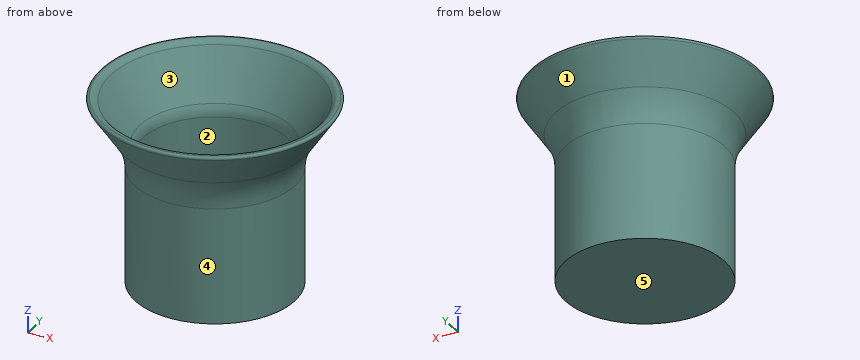
```python
from build123d import *


with BuildPart() as part:
    # Sketch → Revolution (revolve)
    with BuildSketch(Plane.XZ):
        with BuildLine():
            Line((0, 0), (-30, 0))
            Line((-30, 0), (-30, 43.518658))
            ThreePointArc((-30, 43.518658), (-30.926805, 49.716476), (-33.626135, 55.372051))
            Line((-33.626135, 55.372051), (-42.643328, 68.730856))
            ThreePointArc((-41.968787, 70), (-42.687419, 69.568119), (-42.643328, 68.730856))
            Line((-41.968787, 70), (-41.81553, 70))
            ThreePointArc((-39.010557, 68.47778), (-40.219831, 69.594921), (-41.81553, 70))
            Line((-39.010557, 68.47778), (-28.297456, 51.996087))
            ThreePointArc((-27, 47.619295), (-27.331193, 49.901821), (-28.297456, 51.996087))
            Line((-27, 12.91057), (-27, 47.619295))
            ThreePointArc((-27, 12.91057), (-24.243708, 6.256292), (-17.58943, 3.5))
            Line((0, 3.5), (-17.58943, 3.5))
            Line((0, 0), (0, 3.5))
        make_face()
    revolve(axis=Axis((0, 0, 0), (0, 0, 1)))


solid = part.part
```
Part model, mm, in its own coordinate system. Face numbers are marked on the shaded views. A direction names the side the tool comes from. Coordinates: 2 decimals unless noted, no trailing zeros. Order: outer loops, then holes, each group sorted by start corner. A loop starts at its lowest first (then second) coordinate and runs counter-clockwise, first axis right, second up. Notation, with made-up numbers: (28, -6) -> (83, -6) arc R24 ccw to (83, 27) -> close; hole circle Ø1 at (72.5, 41). An arc over 180 degrees is marked (long way). Put each result on its own line as item: value. Start each with the question number.
(1) Band-saw the part on D-D (z = 9.5). Give the cut face in (x, y), then the cut area to 3 significant figures.
(2) Which spindle directions (+Z, -Z, +X, -X, +Y, -Y) get a long thin tool onto all of the face, cutting with end or side? Do the marked faces 1 and 2. Say none if no direction does.
(3) Probe line 1 along X through (y, z) = (0, 25.5); line 2 along Y through (x, z) = (23.5, 65.5). List the from-to ranges inside material, lowest first. Write a range as [from, to].
(4) Band-saw the part on B-B (z = 26). Give the cut face in (x, y), then the cut area to 3 significant figures.
(5) Mould opens along Y. For the marked faces 3, 4 and 5 say: pulls with the +Y half, pulls with the -Y half, needs draft (parallel to the pull), parting line crosses it, or undercut.
(6) Band-saw the part on A-A (x = 0). Give the cut face in (y, z), then the cut area to 3 significant figures.
(7) Pin check, flat tips, straight feed: pin 1 Ø1 at (y, z) = (30, 58.5) entering from -X; pin 2 Ø6 at (x, z) = (-6.5, 45) entering from -Y; pin 3 Ø1 at (y, z) = (-26, 13) entering from +X. Stop position of each tip, or through.
Determined:
1. outline: circle Ø60 at (0, 0); hole circle Ø52.72 at (0, 0)
1. area: 644 mm²
2. face 1: -Z
2. face 2: +Z
3. line 1: x = [-30, -27], [27, 30]
3. line 2: y = [-32.94, -28.68], [28.68, 32.94]
4. outline: circle Ø60 at (0, 0); hole circle Ø54 at (0, 0)
4. area: 537 mm²
5. face 3: undercut
5. face 4: parting line crosses it
5. face 5: needs draft
6. outline: (-42.64, 68.73) -> (-33.63, 55.37) arc R21.19 cw to (-30, 43.52) -> (-30, 0) -> (30, 0) -> (30, 43.52) arc R21.19 cw to (33.63, 55.37) -> (42.64, 68.73) arc R0.81 ccw to (41.97, 70) -> (41.82, 70) arc R3.35 ccw to (39.01, 68.48) -> (28.3, 52) arc R8.03 ccw to (27, 47.62) -> (27, 12.91) arc R9.41 cw to (17.59, 3.5) -> (-17.59, 3.5) arc R9.41 cw to (-27, 12.91) -> (-27, 47.62) arc R8.03 ccw to (-28.3, 52) -> (-39.01, 68.48) arc R3.35 ccw to (-41.82, 70) -> (-41.97, 70) arc R0.81 ccw to start
6. area: 662 mm²
7. pin 1: stops at x = -20.39
7. pin 2: stops at y = -29.99
7. pin 3: stops at x = 15.8
